Autodesk Fusion 360 part; units mm, degrees
sketch "草图1" plane through (0, 0, 0) normal (0, 0, 1) x (1, 0, 0)
  circle A0 centre (-13.6473, 1.2662) radius 16.75
  circle A1 centre (-13.6473, 1.2662) radius 11
  circle A2 centre (3.8527, 20.9662) radius 2
  circle A3 centre (-33.9473, -22.0338) radius 2
  line L0 (10.8527, -25.9797) -> (-13.6473, -25.9797)
  line L1 (-13.6473, -25.9797) -> (-13.6473, 1.2662)
  line L2 (-13.6473, 1.2662) -> (10.8527, 1.2662)
  line L3 (10.8527, 1.2662) -> (10.8527, -25.9797)
  line L4 (10.8527, -25.9797) -> (-39.1473, -25.9797)
  line L5 (-39.1473, -25.9797) -> (-39.1473, 24.0203)
  line L6 (-39.1473, 24.0203) -> (10.8527, 24.0203)
  line L7 (10.8527, 24.0203) -> (10.8527, -25.9797)
  dimension "d1" = 33.5
  dimension "d2" = 22
  dimension "d3" = 19.7
  dimension "d4" = 17.5
  dimension "d5" = 4
  dimension "d6" = 20.3
  dimension "d7" = 23.3
  dimension "d8" = 4
  dimension "d9" = 24.5
  dimension "d11" = 50
  dimension "d12" = 50
sketch "草图2" plane through (0, 0, 0) normal (0, 0, 1) x (1, 0, 0)
  line L0 (10.8527, 24.0203) -> (10.8527, -25.9797)
  line L1 (-39.1473, 24.0203) -> (10.8527, 24.0203)
  line L2 (-39.1473, -25.9797) -> (-39.1473, 24.0203)
  line L3 (10.8527, -25.9797) -> (-39.1473, -25.9797)
  line L4 (-13.6473, 1.2662) -> (-13.6473, 24.0203) construction
  line L5 (-13.6473, 1.2662) -> (10.8527, 1.2662) construction
  line L6 (-13.6473, 1.2662) -> (-39.1473, 1.2662) construction
  line L7 (-39.1473, 1.2662) -> (-13.6473, 1.2662)
  line L8 (-13.6473, -25.9797) -> (-13.6473, 1.2662) construction
  ellipse E0 centre (-13.6473, 1.2662) end of major axis (-13.6473, 24.0203) minor radius 21.4054 (7.7581, 1.2662) -> (-13.6473, 24.0203) ccw
  ellipse E1 centre (-13.6473, 1.2662) end of major axis (-13.6473, 24.0203) minor radius 25.5 (-13.6473, 24.0203) -> (-39.1473, 1.2662) ccw
  ellipse E2 centre (-13.6473, 1.2662) end of major axis (-39.1473, 1.2662) minor radius 27.2458 (-39.1473, 1.2662) -> (-13.6473, -25.9797) ccw
  line L9 (10.8527, 1.2662) -> (7.7581, 1.2662)
  point P0 (-13.6473, 1.2662)
extrude "拉伸1" add sketch "草图2" against normal blind 20 contours L0 L3 E0 E1 E2 L9
sketch "草图3" plane through (10.8527, 0, 0) normal (1, 0, 0) x (0, 1, 0)
  line L0 (1.2662, 0) -> (-25.9797, 0)
  line L1 (-25.9797, 0) -> (-25.9797, -20)
  line L2 (-25.9797, -20) -> (1.2662, -20)
  line L3 (1.2662, -20) -> (1.2662, 0)
  line L4 (-24.0386, -1.9) -> (-1.3386, -1.9)
  line L5 (-1.3386, -1.9) -> (-1.3386, -18.1)
  line L6 (-1.3386, -18.1) -> (-24.0386, -18.1)
  line L7 (-24.0386, -18.1) -> (-24.0386, -1.9)
  point P0 (-1.3386, -10)
  point P1 (1.2662, -10)
  point P2 (-12.3567, 0)
  point P3 (-12.6886, -1.9)
  dimension "d15" = 22.7
  dimension "d16" = 16.2
extrude "拉伸2" cut sketch "草图3" against normal blind 5 contours L4 L5 L6 L7
For this review, take the finished solid that the model builds, in its own axes (mm). A direction names the side the tool comes from. Give positions to 0.01 mm unless a question says otherwise; leave off trailing zeros. One line per item, written item: value.
1) For line 1 (Y direction, x = -17, z = -4.75); line 2 (Y direction, x = -16, z = -18.75); line 3 (X direction, y = 16, z = -14), list the stretches that pass through material, from the lowest coordinate up. Write a range as from..to.
Results are:
line 1: y = -25.74..23.82
line 2: y = -25.86..23.92
line 3: x = -33.08..2.66
2) The part is to be moulded in two halves that separate along Z. For faces 4 (the flat face through (5.853, -13, -10)), 5 (the flat face through (-14, -1, 0)), 6 (the flat face through (10.853, -12, -19)), say which applies: +Z half, -Z half, draft (parallel to the pull), parting line (faces both ways), or undercut.
Results are:
face 4: undercut
face 5: +Z half
face 6: draft
3) For faces 1 (the flat face through (8, -1.339, -10)), 2 (the flat face through (-1, -25.98, -10)), 3 (the flat face through (9, 1.266, -10)), list the 3-axis set-ups (+Z, -Z, +X, -X, +Y, -Y) from which the entire face can be reached by the end or side of a thin tool; tool diameter is ignored.
Results are:
face 1: +X
face 2: +Z, -Z, +X, -X, -Y
face 3: +Z, -Z, +X, +Y
4) For P1, Ø12, axis at x = -33.5, z = -13, coming from the +Y side; P2, Ø2.5, axis at x = 9.5, z = -9.5, coming from the +Y side; P3, Ø8, axis at x = -18, z = -6.5, coming from the -Y side, all flat-tipped, find the tip position at first contact; note any pin that passes through.
Results are:
P1: stops at y = 20.37
P2: stops at y = 1.27
P3: stops at y = -25.98
